from build123d import *

# Parameters (mm, degrees)
BOSS_EXTRUDE1_DEPTH     = 250
BOSS_EXTRUDE2_START     = -167
BOSS_EXTRUDE2_DEPTH     = 167
CUT_EXTRUDE1_REACH      = 314.698
CUT_EXTRUDE1_END_RADIUS = 28.575
BOSS_EXTRUDE3_START     = 33
BOSS_EXTRUDE3_DEPTH     = 33
CUT_EXTRUDE2_DEPTH      = 13


with BuildPart() as part:
    # Sketch1 → Boss-Extrude1 (new body)
    with BuildSketch(Plane.XY):
        with BuildLine():
            Line((-84, 0), (-84, -43.008130888))
            Line((-84, -43.008130888), (-13, -84))
            Line((-13, -84), (0, -84))
            Line((0, -84), (0, -44.45))
            ThreePointArc((0, -44.45), (-44.45, 0), (0, 44.45))
            Line((0, 44.45), (0, 84))
            ThreePointArc((0, 84), (-59.39696962, 59.39696962), (-84, 0))
        make_face()
    extrude(amount=-BOSS_EXTRUDE1_DEPTH)

    # Sketch2 → Boss-Extrude2 (add)
    with BuildSketch(Plane(origin=(0, 0, -250), x_dir=(-1, 0, 0), z_dir=(0, 0, -1)).offset(BOSS_EXTRUDE2_START)):
        with BuildLine():
            Line((0, 28.575), (0, 44.45))
            ThreePointArc((0, 44.45), (44.45, 0), (0, -44.45))
            Line((0, -44.45), (0, -28.575))
            ThreePointArc((0, -28.575), (28.575, 0), (0, 28.575))
        make_face()
    extrude(amount=BOSS_EXTRUDE2_DEPTH)

    # Cut-Extrude1: up to this cylinder (the profile starts outside it)
    cut_extrude1_end = Plane(origin=(0, 0, -195.5), z_dir=(0, 0, -1)) * Cylinder(CUT_EXTRUDE1_END_RADIUS, 687.546, mode=Mode.PRIVATE)
    # Sketch3 → Cut-Extrude1 (cut, up to the surface)
    with BuildSketch(Plane(origin=(0, 84, 0), x_dir=(1, 0, 0), z_dir=(0, 1, 0)), mode=Mode.PRIVATE) as cut_extrude1_sk1:
        Polygon((0, 179), (0, 212), (-19, 210.337715393), (-19, 180.662284607), align=None)
    cut_extrude1_tool1 = extrude(cut_extrude1_sk1.sketch, amount=-CUT_EXTRUDE1_REACH, mode=Mode.PRIVATE) - cut_extrude1_end
    add(cut_extrude1_tool1.solids().sort_by_distance((-9.332027, 84, -195.5))[0], mode=Mode.SUBTRACT)

    # Sketch4 → Boss-Extrude3 (add)
    with BuildSketch(Plane.XY.offset(BOSS_EXTRUDE3_START)):
        with BuildLine():
            Line((-83.014649379, 12.828405531), (-65.430668922, -0.909705656))
            Line((-65.430668922, -0.909705656), (-14.946427946, 63.707176139))
            Line((-14.946427946, 63.707176139), (-32.530408402, 77.445287327))
            ThreePointArc((-32.530408402, 77.445287327), (-66.192903303, 51.715563927), (-83.014649379, 12.828405531))
        make_face()
    extrude(amount=-BOSS_EXTRUDE3_DEPTH)

    # Sketch5 → Cut-Extrude2 (cut)
    with BuildSketch(Plane(origin=(0, 0, 0), x_dir=(0, 0, -1), z_dir=(1, 0, 0))):
        with BuildLine():
            Line((250, -69), (133, -69))
            ThreePointArc((133, -69), (122, -58), (133, -47))
            Line((133, -47), (250, -47))
            ThreePointArc((250, -47), (261, -58), (250, -69))
        make_face()
    extrude(amount=-CUT_EXTRUDE2_DEPTH, mode=Mode.SUBTRACT)


solid = part.part
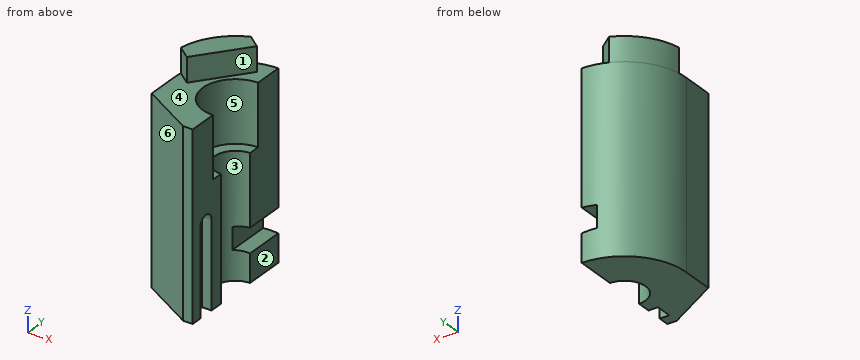
Geometry: final body of the model. Coordinates: model frame, mm. Face numbers are marked on the shaded views. A direction names the side the tool comes from. Coordinates: 2 decimals unless noted, no trailing zeros. Write each loop counter-clockwise with the first axis right and the second up, starting at its lowest first coordinate (ties: lowest second). Pieces come first, ordered by that corner, then holes. Notation, with made-up numbers: (50, 49) - (88, 49) arc R22 cw to (88, 56) - close; hole circle Ø7 at (-37.75, 17). An arc over 180 degrees is marked (long way). Return JSON: item names as keys, results as strings.
Item 1: Section query D-D (y = 39). Output: boundary loops of the cut face in (x, z).
Completed:
{"outline": "(-74.4, -250) - (0, -250) - (0, -212) - (-19, -210.34) - (-19, -180.66) - (0, -179) - (0, -83) - (-21.33, -83) - (-21.33, 0) - (-34.25, 0) - (-34.25, 33) - (-74.4, 33) - close"}
Item 2: Pull-direction query (Y, two-part tool) for the marked faces 3, 4, 5 and 6; classes: +Y half, -Y half, draft (parallel to the pull), parting line (faces both ways), or undercut.
Completed:
{"face 3": "undercut", "face 4": "draft", "face 5": "undercut", "face 6": "-Y half"}
Item 3: Pin query (flat end, axial travel): pin 1 Ø22 at (x, y) = (-24.5, 9) entering from +Z; pin 2 Ø10 at (y, z) = (26.5, -16) entering from +X; pin 3 Ø4 at (x, z) = (-19, -159) entering from +Y. Return the tip coordinate at first contact, or that it passes through.
Completed:
{"pin 1": "stops at z = -83", "pin 2": "stops at x = -31.36", "pin 3": "stops at y = 82.26"}
Item 4: Line query: L1, parallel to Y at x = -7, z = -154; L2, parallel to Z at x = -72, y = -7.5; L3, parallel to Y at x = -32, z = -35.5. Output: solid intervals per line, ascending.
Completed:
{"L1": "y = -84 to -69, -47 to -27.7, 27.7 to 83.71", "L2": "z = -250 to 0", "L3": "y = -73.03 to -30.85, 30.85 to 77.67"}
Item 5: Reachability of the marked faces 1 and 2 from +Z, -Z, +X, -X, +Y, -Y: full face, straight path, thin tool, end or side. Return the list, or none.
Completed:
{"face 1": "+Z, +X, -Y", "face 2": "+Z, -Z, +X, +Y, -Y"}
Item 6: Section query C-C (x = -5.5). Output: boundary loops of the cut face in (y, z).
Completed:
{"outline": "(-84, -250) - (-69, -250) - (-69, -133) arc R11 cw to (-47, -133) - (-47, -250) - (-28.04, -250) - (-28.04, -83) - (-44.11, -83) - (-44.11, 0) - (-84, 0) - close; (28.04, -250) - (83.82, -250) - (83.82, -211.52) - (28.04, -211.52) - close; (28.04, -179.48) - (83.82, -179.48) - (83.82, 0) - (44.11, 0) - (44.11, -83) - (28.04, -83) - close"}
Item 7: Section query A-A (z = -46). Output: boundary loops of the cut face in (x, y), and give its area (3 significant figures).
Completed:
{"outline": "(-84, -43.01) - (-13, -84) - (0, -84) - (0, -44.45) arc R44.45 cw to (0, 44.45) - (0, 84) arc R84 ccw to (-84, 0) - close", "area": "8,040 mm2"}
Item 8: Section query B-B (x = -22). Output: boundary loops of the cut face in (y, z).
Completed:
{"outline": "(-78.8, -250) - (-18.24, -250) - (-18.24, -83) - (-38.62, -83) - (-38.62, 0) - (-78.8, 0) - close; (18.24, -250) - (81.07, -250) - (81.07, 0) - (69.22, 0) - (69.22, 33) - (54.68, 33) - (54.68, 0) - (38.62, 0) - (38.62, -83) - (18.24, -83) - close"}
